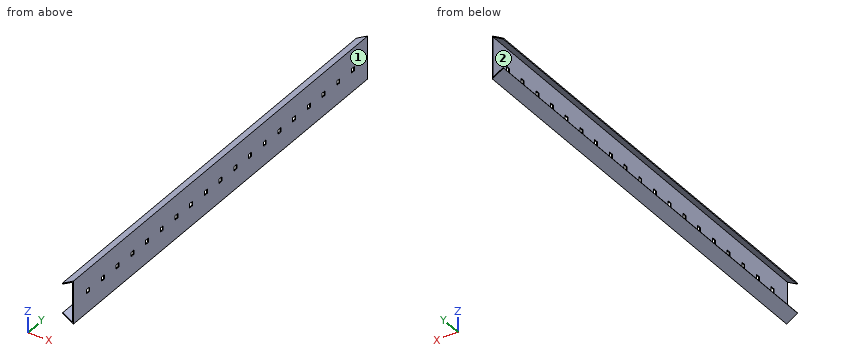
Autodesk Inventor part; units mm, degrees
ref_plane "YZ Plane" through (0, 0, 0) normal (1, 0, 0) x (0, 1, 0)
ref_plane "XZ Plane" through (0, 0, 0) normal (0, 1, 0) x (-1, 0, 0)
ref_plane "XY Plane" through (0, 0, 0) normal (0, 0, 1) x (1, 0, 0)
sketch "Sketch1" plane through (0, 0, 0) normal (0, 1, 0) x (-1, 0, 0)
  line L0 (0, 0) -> (0, 12.7)
  line L1 (0, 12.7) -> (3.2996, 10.795)
  line L2 (0, 0) -> (3.2996, 1.905)
  line L3 (0, 0) -> (3.81, 0) construction
  line L4 (3.1726, 10.575) -> (0.254, 12.2601)
  line L5 (0.254, 12.2601) -> (0.254, 0.4399)
  line L6 (0.254, 0.4399) -> (3.1726, 2.125)
  line L7 (3.1726, 10.575) -> (3.2996, 10.795)
  line L8 (3.1726, 2.125) -> (3.2996, 1.905)
  dimension "d0" = 12.7
  dimension "d1" = 3.81
  dimension "d2" = 60
  dimension "d3" = 30
  dimension "d4" = 0.254
extrude "Extrusion1" add sketch "Sketch1" along normal blind 127
sketch "Sketch2" plane through (-0.254, 0, 0.4399) normal (-1, 0, 0) x (0, 0, 1)
  line L0 (5.2751, 5.715) -> (6.5451, 5.715)
  line L1 (6.5451, 5.715) -> (6.5451, 6.985)
  line L2 (6.5451, 6.985) -> (5.2751, 6.985)
  line L3 (5.2751, 6.985) -> (5.2751, 5.715)
  line L4 (5.2751, 5.715) -> (6.5451, 6.985) construction
  line L5 (6.5451, 5.715) -> (5.2751, 6.985) construction
  line L6 (6.5451, 12.065) -> (6.5451, 13.335)
  line L7 (6.5451, 13.335) -> (5.2751, 13.335)
  line L8 (5.2751, 13.335) -> (5.2751, 12.065)
  line L9 (5.2751, 12.065) -> (6.5451, 12.065)
  line L10 (6.5451, 18.415) -> (6.5451, 19.685)
  line L11 (6.5451, 19.685) -> (5.2751, 19.685)
  line L12 (5.2751, 19.685) -> (5.2751, 18.415)
  line L13 (5.2751, 18.415) -> (6.5451, 18.415)
  line L14 (6.5451, 24.765) -> (6.5451, 26.035)
  line L15 (6.5451, 26.035) -> (5.2751, 26.035)
  line L16 (5.2751, 26.035) -> (5.2751, 24.765)
  line L17 (5.2751, 24.765) -> (6.5451, 24.765)
  line L18 (6.5451, 31.115) -> (6.5451, 32.385)
  line L19 (6.5451, 32.385) -> (5.2751, 32.385)
  line L20 (5.2751, 32.385) -> (5.2751, 31.115)
  line L21 (5.2751, 31.115) -> (6.5451, 31.115)
  line L22 (6.5451, 37.465) -> (6.5451, 38.735)
  line L23 (6.5451, 38.735) -> (5.2751, 38.735)
  line L24 (5.2751, 38.735) -> (5.2751, 37.465)
  line L25 (5.2751, 37.465) -> (6.5451, 37.465)
  line L26 (6.5451, 43.815) -> (6.5451, 45.085)
  line L27 (6.5451, 45.085) -> (5.2751, 45.085)
  line L28 (5.2751, 45.085) -> (5.2751, 43.815)
  line L29 (5.2751, 43.815) -> (6.5451, 43.815)
  line L30 (6.5451, 50.165) -> (6.5451, 51.435)
  line L31 (6.5451, 51.435) -> (5.2751, 51.435)
  line L32 (5.2751, 51.435) -> (5.2751, 50.165)
  line L33 (5.2751, 50.165) -> (6.5451, 50.165)
  line L34 (6.5451, 56.515) -> (6.5451, 57.785)
  line L35 (6.5451, 57.785) -> (5.2751, 57.785)
  line L36 (5.2751, 57.785) -> (5.2751, 56.515)
  line L37 (5.2751, 56.515) -> (6.5451, 56.515)
  line L38 (6.5451, 62.865) -> (6.5451, 64.135)
  line L39 (6.5451, 64.135) -> (5.2751, 64.135)
  line L40 (5.2751, 64.135) -> (5.2751, 62.865)
  line L41 (5.2751, 62.865) -> (6.5451, 62.865)
  line L42 (6.5451, 69.215) -> (6.5451, 70.485)
  line L43 (6.5451, 70.485) -> (5.2751, 70.485)
  line L44 (5.2751, 70.485) -> (5.2751, 69.215)
  line L45 (5.2751, 69.215) -> (6.5451, 69.215)
  line L46 (6.5451, 75.565) -> (6.5451, 76.835)
  line L47 (6.5451, 76.835) -> (5.2751, 76.835)
  line L48 (5.2751, 76.835) -> (5.2751, 75.565)
  line L49 (5.2751, 75.565) -> (6.5451, 75.565)
  line L50 (6.5451, 81.915) -> (6.5451, 83.185)
  line L51 (6.5451, 83.185) -> (5.2751, 83.185)
  line L52 (5.2751, 83.185) -> (5.2751, 81.915)
  line L53 (5.2751, 81.915) -> (6.5451, 81.915)
  line L54 (6.5451, 88.265) -> (6.5451, 89.535)
  line L55 (6.5451, 89.535) -> (5.2751, 89.535)
  line L56 (5.2751, 89.535) -> (5.2751, 88.265)
  line L57 (5.2751, 88.265) -> (6.5451, 88.265)
  line L58 (6.5451, 94.615) -> (6.5451, 95.885)
  line L59 (6.5451, 95.885) -> (5.2751, 95.885)
  line L60 (5.2751, 95.885) -> (5.2751, 94.615)
  line L61 (5.2751, 94.615) -> (6.5451, 94.615)
  line L62 (6.5451, 100.965) -> (6.5451, 102.235)
  line L63 (6.5451, 102.235) -> (5.2751, 102.235)
  line L64 (5.2751, 102.235) -> (5.2751, 100.965)
  line L65 (5.2751, 100.965) -> (6.5451, 100.965)
  line L66 (6.5451, 107.315) -> (6.5451, 108.585)
  line L67 (6.5451, 108.585) -> (5.2751, 108.585)
  line L68 (5.2751, 108.585) -> (5.2751, 107.315)
  line L69 (5.2751, 107.315) -> (6.5451, 107.315)
  line L70 (6.5451, 113.665) -> (6.5451, 114.935)
  line L71 (6.5451, 114.935) -> (5.2751, 114.935)
  line L72 (5.2751, 114.935) -> (5.2751, 113.665)
  line L73 (5.2751, 113.665) -> (6.5451, 113.665)
  line L74 (6.5451, 120.015) -> (6.5451, 121.285)
  line L75 (6.5451, 121.285) -> (5.2751, 121.285)
  line L76 (5.2751, 121.285) -> (5.2751, 120.015)
  line L77 (5.2751, 120.015) -> (6.5451, 120.015)
  point P0 (-0.4399, 0)
  point P1 (5.9101, 6.35)
  dimension "d7" = 1.27
  dimension "d8" = 1.27
  dimension "d14" = 6.35
extrude "Extrusion2" cut sketch "Sketch2" against normal blind 0.254
properties part number "Thing1"
The model under review builds one solid part; all positions refer to its coordinate system, in mm. Face numbers are marked on the shaded views. Give positions to 0.01 mm unless a question says otherwise; leave off trailing zeros. Write each loop counter-clockwise with the first axis right and the second up, starting at its lowest first coordinate (ties: lowest second). Pieces come first, ordered by that corner, then holes. Notation, with made-up numbers: M -33.75,81 L -11.75,81 A18 ccw -11.75,88 Z; hole C -17,62 d1. An arc over 180 degrees is marked long. Write each question's results on one line, items separated by ' | '. Start each with the question number.
1. Mouldability with a two-part tool opening along Z and no side actions: class the marked faces 1 and 2 as released by +Z, released by -Z, zero draft, split by the parting line, or undercut.
2. For probe 1 along X at (y, z) = (55.5, 7); probe 2 along Z at (x, y) = (-1.75, 110.5); probe 3 along Z at (x, y) = (-0.7, 112), list the stretches that pass through material, from the lowest coordinate up. Write a range as [from, to].
3. We need section C-C (z = 9.5). Write out the cut boundary in (x, y), and give its area (3 significant figures).
4. We need section A-A (x = -2.3). Write out the cut boundary in (y, z).
5. Insertion check: pin 1 Ø5 at (y, z) = (93.5, 7) entering from -X; pin 2 Ø1 at (x, z) = (-1.5, 8) entering from +Y. Each pin has a flat end and moves straight along its axis. Give the tip position at first contact, or say it passes through.
6. We need section B-B (y = 98). Write out the cut boundary in (x, z) (3 decimals).
Results found:
1) face 1: zero draft | face 2: undercut
2) probe 1: x = [-0.25, 0] | probe 2: z = [1.01, 1.3], [11.4, 11.69] | probe 3: z = [0.4, 0.7], [12, 12.3]
3) outline: M -0.25,0 L 0,0 L 0,127 L -0.25,127 Z | area: 32.3 mm^2
4) outline: M 0,1.33 L 127,1.33 L 127,1.62 L 0,1.62 Z; M 0,11.08 L 127,11.08 L 127,11.37 L 0,11.37 Z
5) pin 1: stops at x = -0.25 | pin 2: passes through
6) outline: M -3.3,1.905 L 0,0 L 0,12.7 L -3.3,10.795 L -3.173,10.575 L -0.254,12.26 L -0.254,0.44 L -3.173,2.125 Z
